Design review of the part built by this model. Coordinates are the model's own, in mm. Face numbers are marked on the shaded views. A direction names the side the tool comes from. Coordinates: 2 decimals unless noted, no trailing zeros. Loops run counter-clockwise (first coordinate to the right, second up) from the corner with the lowest first, then second, coordinate; pieces in that order, holes last. Notation, with made-up numbers: (25.5, 21.25) -> (35.5, 21.25) arc R10 cw to (35.5, 37.25) -> close; hole circle Ø1 at (27.25, -23). An arc over 180 degrees is marked (long way). One line per item, written item: value. Start each with the question number.
1. Add section A-A on z = -8. Write out the cut boundary in (x, y).
2. Machinability: for the marked faces 1, 2 and 3, which of the approach directions +Z, -Z, +X, -X, +Y, -Y give a long, thin tool a straight path to every point of the face, cutting with its end or side? Answer none if there is none.
3. For probe 1 along X at (y, z) = (9.75, -25); probe 2 along X at (y, z) = (3.5, 17); probe 3 along Z at (x, y) = (1, 7.75), list the stretches that pass through material, from the lowest coordinate up.
4. Add section C-C on y = 8. Write out the cut boundary in (x, z).
5. Add section D-D on z = 9.5. Write out the cut boundary in (x, y).
6. Insertion check: pin 1 (3.5 mm diameter, centred on x = -10.5, z = -27.5, fed in from -Y); pin 2 (0.9 mm diameter, centred on x = 14, z = -26.5, fed in from -Y); pin 3 (8 mm diameter, centred on x = -6.5, z = -15, fed in from +Y); pin 4 (10 mm diameter, centred on x = -4.5, z = 0, fed in from -Y). Each pin has a flat end and moves straight along its axis. Give the tip position at first contact, or say it passes through.
7. Draft analysis for pull direction X (two halves, no side actions). For the marked faces 4, 5, 6 and 7, state which applies: pulls with the +X half, pulls with the -X half, needs draft (parallel to the pull), parting line crosses it, or undercut.
Autodesk Inventor part; units mm, degrees
ref_plane "YZ Plane" through (0, 0, 0) normal (1, 0, 0) x (0, 1, 0)
ref_plane "XZ Plane" through (0, 0, 0) normal (0, 1, 0) x (-1, 0, 0)
ref_plane "XY Plane" through (0, 0, 0) normal (0, 0, 1) x (1, 0, 0)
sketch "Sketch1" plane through (0, 0, 0) normal (0, 1, 0) x (-1, 0, 0)
  line L0 (-1.5171, 15.4904) -> (-1.5171, -24.1277) construction
  line L1 (12.4829, 23.2632) -> (-15.5171, 23.2632)
  line L2 (-15.5171, 23.2632) -> (-15.5171, -31.7368)
  line L3 (-15.5171, -31.7368) -> (12.4829, -31.7368)
  line L4 (12.4829, -31.7368) -> (12.4829, 23.2632)
  line L5 (1.173, -11.7368) -> (-5.6801, -11.7368) construction
  circle A0 centre (-1.5171, -11.7368) radius 11
  line L6 (8.4829, 8.2632) -> (-11.5171, 8.2632)
  line L7 (-11.5171, 8.2632) -> (-11.5171, 23.2632)
  line L8 (-11.5171, 23.2632) -> (8.4829, 23.2632)
  line L9 (8.4829, 23.2632) -> (8.4829, 8.2632)
  point P0 (0, 0)
  dimension "d0" = 22
  dimension "d1" = 28
  dimension "d2" = 20
  dimension "d3" = 15
  dimension "d4" = 20
  dimension "d16" = 55
extrude "Extrusion1" add sketch "Sketch1" along normal blind 10 contours L4 L3 L2 L1 L7 L6 L9
extrude "Extrusion2" add sketch "Sketch1" along normal blind 6.4 contours A0
sketch "Sketch2" plane through (0, 10, 0) normal (0, 1, 0) x (1, 0, 0)
  line L0 (11.5171, -8.2632) -> (-8.4829, -8.2632)
  line L1 (-8.4829, -8.2632) -> (11.5171, -8.2632)
  line L2 (11.5171, -8.2632) -> (11.5171, -18.2632)
  line L3 (11.5171, -18.2632) -> (-8.4829, -18.2632)
  line L4 (-8.4829, -18.2632) -> (-8.4829, -8.2632)
  point P0 (0, 0)
  dimension "d9" = 10
extrude "Extrusion3" add sketch "Sketch2" against normal blind 5
sketch "Sketch3" plane through (15.5171, 0, 23.2632) normal (1, 0, 0) x (0, 0, -1)
  line L0 (0, 0) -> (55, 0) construction
  line L1 (55, 0) -> (55, 10) construction
  line L2 (0, 10) -> (55, 10) construction
  line L3 (0, 0) -> (0, 10) construction
  line L4 (55, 0) -> (19, 0)
  line L5 (19, 0) -> (19, 4)
  line L6 (19, 4) -> (55, 4)
  line L7 (55, 4) -> (55, 0)
  line L8 (24, 6.4) -> (46, 6.4) construction
  line L9 (24, 10) -> (46, 10) construction
  point P0 (23.2632, 0)
  dimension "d12" = 6
  dimension "d17" = 5
extrude "Extrusion4" cut sketch "Sketch3" against normal through all
sketch "Sketch4" plane through (15.5171, 4, -31.7368) normal (0, -1, 0) x (1, 0, 0)
  line L0 (1.7907, 5) -> (-31.4365, 5) construction
  line L1 (0, 0) -> (-28, 0) construction
  line L2 (-3, 7) -> (-7, 7)
  line L3 (-7, 7) -> (-7, 3)
  line L4 (-7, 3) -> (-3, 3)
  line L5 (-3, 3) -> (-3, 7)
  line L6 (-5, 9.5929) -> (-5, 0.7775) construction
  line L7 (0, 36) -> (0, 0) construction
  line L8 (-14, 47.2272) -> (-14, 7.6092) construction
  line L9 (-25, 7) -> (-21, 7)
  line L10 (-21, 7) -> (-21, 3)
  line L11 (-21, 3) -> (-25, 3)
  line L12 (-25, 3) -> (-25, 7)
  point P0 (-15.5171, 31.7368)
  dimension "d18" = 5
  dimension "d19" = 4
  dimension "d20" = 5
extrude "Extrusion5" cut sketch "Sketch4" against normal through all
fillet "Fillet1" radius 2 2 edges at (1.5171, 4, 4.2632) (1.5171, 0, 4.2632)
sketch "Sketch5" plane through (0, 10, 0) normal (0, 1, 0) x (1, 0, 0)
  line L0 (11.5171, -18.2632) -> (-8.4829, -18.2632) construction
  line L1 (1.5171, -18.2632) -> (1.5171, -0.9417) construction
  circle A0 centre (1.5171, -13.2632) radius 1.5
  point P0 (0, 0)
  dimension "d24" = 3
  dimension "d25" = 5
extrude "Extrusion6" cut sketch "Sketch5" against normal through all
sketch "Sketch6" plane through (1.5171, 6.4, -11.7368) normal (0, 1, 0) x (1, 0, 0)
  circle A0 centre (0, 0) radius 11 construction
  circle A1 centre (0, 0) radius 8
  point P0 (-1.5171, -11.7368)
  dimension "d28" = 3
extrude "Extrusion7" cut sketch "Sketch6" against normal through all
sketch "Sketch8" plane through (-12.4829, 4, -31.7368) normal (0, -1, 0) x (1, 0, 0)
  circle A0 centre (14, 20) radius 8 construction
  line L0 (0, 34) -> (28, 34) construction
  line L1 (0, 0) -> (0, 34) construction
  line L2 (28, 0) -> (0, 0) construction
  line L3 (28, 34) -> (28, 0) construction
  line L4 (21, 3) -> (21, 7) construction
  line L5 (21, 7) -> (25, 7) construction
  line L6 (25, 7) -> (25, 3) construction
  line L7 (25, 3) -> (21, 3) construction
  line L8 (3, 3) -> (3, 7) construction
  line L9 (3, 7) -> (7, 7) construction
  line L10 (7, 7) -> (7, 3) construction
  line L11 (7, 3) -> (3, 3) construction
  line L12 (3, 7) -> (-3.7941, 7)
  line L13 (-3.7941, 7) -> (-3.7941, 3)
  line L14 (-3.7941, 3) -> (3, 3)
  line L15 (3, 3) -> (3, 7)
  line L16 (25, 7) -> (32.0495, 7)
  line L17 (32.0495, 7) -> (32.0495, 3)
  line L18 (32.0495, 3) -> (25, 3)
  line L19 (25, 3) -> (25, 7)
  point P0 (12.4829, 31.7368)
extrude "Extrusion9" cut sketch "Sketch8" against normal blind 2
properties part number "PISTON_bearing"
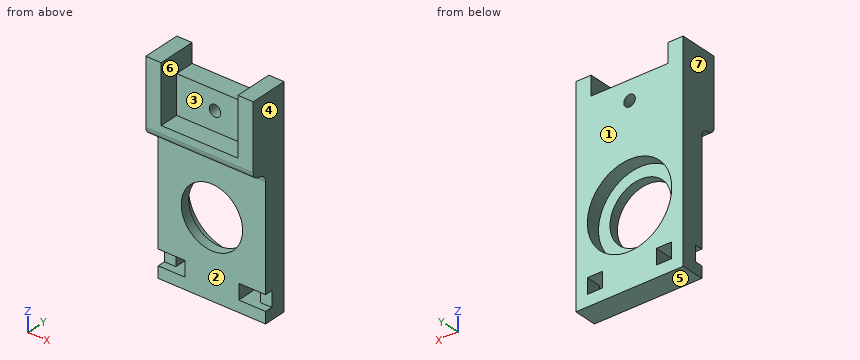
Worked answers:
1. outline: (-12.48, 4) -> (-5.56, 4) -> (-5.56, 6.4) -> (-8.83, 6.4) -> (-8.83, 10) -> (-12.48, 10) -> close; (8.59, 4) -> (15.52, 4) -> (15.52, 10) -> (11.86, 10) -> (11.86, 6.4) -> (8.59, 6.4) -> close
2. face 1: +Z, -Z, +X, -X, +Y
2. face 2: -Z, +X, -X, -Y
2. face 3: +Z, -Y
3. probe 1: x = -12.48 to -9.48, -5.48 to 8.52, 12.52 to 15.52
3. probe 2: x = -12.48 to -8.48, 11.52 to 15.52
3. probe 3: z = -31.74 to -22.72, -0.75 to 11.86, 14.67 to 18.26
4. outline: (-12.48, -31.74) -> (15.52, -31.74) -> (15.52, 23.26) -> (11.52, 23.26) -> (11.52, 18.26) -> (-8.48, 18.26) -> (-8.48, 23.26) -> (-12.48, 23.26) -> close; hole (-9.48, -28.74) -> (-5.48, -28.74) -> (-5.48, -24.74) -> (-9.48, -24.74) -> close; hole circle Ø22 at (1.52, -11.74); hole circle Ø3 at (1.52, 13.26); hole (8.52, -28.74) -> (12.52, -28.74) -> (12.52, -24.74) -> (8.52, -24.74) -> close
5. outline: (-12.48, 0) -> (-8.48, 0) -> (-8.48, 5) -> (11.52, 5) -> (11.52, 0) -> (15.52, 0) -> (15.52, 10) -> (-12.48, 10) -> close
6. pin 1: stops at y = 4
6. pin 2: stops at y = 6
6. pin 3: stops at y = 10
6. pin 4: stops at y = 0.45
7. face 4: pulls with the +X half
7. face 5: needs draft
7. face 6: undercut
7. face 7: pulls with the -X half
